from build123d import *

# Parameters (mm, degrees)
EXTRUDE_1_DEPTH     = 310
SKETCH_2_R          = 2.2
CUT_EXTRUDE_1_DEPTH = 310
SKETCH_3_R          = 2.2
CUT_EXTRUDE_2_DEPTH = 160


with BuildPart() as part:
    # ｽｹｯﾁ1 → ﾎﾞｽ - 押し出し1 (new body)
    with BuildSketch(Plane.XY):
        Polygon((0, 0), (0, -15), (15, -15), (15, -13.5), (1.5, -13.5), (1.5, 0), align=None)
    extrude(amount=EXTRUDE_1_DEPTH)

    # ｽｹｯﾁ2 → ｶｯﾄ - 押し出し1 (cut)
    with BuildSketch(Plane.ZY):
        with Locations((248, -7.5)):
            Circle(SKETCH_2_R)
        with Locations((186, -7.5)):
            Circle(SKETCH_2_R)
        with Locations((124, -7.5)):
            Circle(SKETCH_2_R)
        with Locations((62, -7.5)):
            Circle(SKETCH_2_R)
    extrude(amount=-CUT_EXTRUDE_1_DEPTH, mode=Mode.SUBTRACT)

    # ｽｹｯﾁ3 → ｶｯﾄ - 押し出し2 (cut)
    with BuildSketch(Plane(origin=(0, -15, 0), x_dir=(-1, 0, 0), z_dir=(0, -1, 0))):
        with Locations((-7.5, -265)):
            Circle(SKETCH_3_R)
        with Locations((-7.5, -155)):
            Circle(SKETCH_3_R)
        with Locations((-7.5, -45)):
            Circle(SKETCH_3_R)
    extrude(amount=-CUT_EXTRUDE_2_DEPTH, mode=Mode.SUBTRACT)


solid = part.part
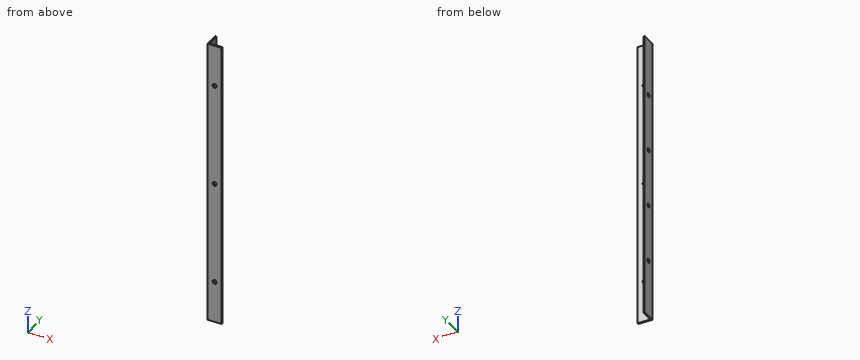
Design review of the part built by this model. Coordinates are the model's own, in mm. Coordinates: 2 decimals unless noted, no trailing zeros. Loops run counter-clockwise (first coordinate to the right, second up) from the corner with the lowest first, then second, coordinate; pieces in that order, holes last. Notation, with made-up numbers: M 1.25,51 L 14.25,51 A26 cw 14.25,88 Z; hole C 53.25,14.5 d2. An arc over 180 degrees is marked long. Use one line per item in the form item = value.
(1) For line 1 along Z through (x, y) = (7.5, -14.6); line 2 along Y through (x, z) = (0.75, 186); line 3 along Y through (x, z) = (14.25, 19.5), list the stretches that pass through material, from the lowest coordinate up. Write a range as from..to.
Return value:
line_1 = 0..42.8, 47.2..152.8, 157.2..262.8, 267.2..310
line_2 = -15..-9.7, -5.3..0
line_3 = -15..-13.5
(2) Clearance check with flat-ended pins moving along their axes: P1, Ø7, axis at y = -4.5, z = 222.5, coming from the +X side; P2, Ø4, axis at x = 5, y = -13, coming from the +Z side; P3, Ø4, axis at x = 10.5, z = 89.5, coming from the +Y side. State where each tip first meets the part, or that it passes through.
Return value:
P1 = 1.5
P2 = 310
P3 = -13.5
(3) Consider section B-B (y = -2.25). Write out the cut boundary in (x, z), and give its area (3 significant figures).
Return value:
outline = M 0,0 L 1.5,0 L 1.5,310 L 0,310 Z
area = 465 mm2
(4) Consider section A-A (z = 226.5). Write out the cut boundary in (x, y), and give its area (4 significant figures).
Return value:
outline = M 0,-15 L 15,-15 L 15,-13.5 L 1.5,-13.5 L 1.5,0 L 0,0 Z
area = 42.75 mm2
